Read the model definition and answer for the solid it produces. Units are mm, in the model's axes. A direction names the side the tool comes from. Coordinates: 2 decimals unless noted, no trailing zeros. Loops run counter-clockwise (first coordinate to the right, second up) from the corner with the lowest first, then second, coordinate; pieces in that order, holes last. Notation, with made-up numbers: M -38,8.25 L 5,8.25 A15 ccw 5,33.25 Z; hole C 30,85.25 d7. An arc over 180 degrees is marked long. Use one line per item in the form item = value. Start each with the question number.
1. For a pull along Z with two mould halves and no side action, classify faces 3 (the flat face through (0, 2, 8.334)), 4 (the cylindrical face through (0.628, 1.565, -14.274)), 5 (the flat face through (6, 0, 3)) as released by +Z, released by -Z, zero draft, split by the parting line, or undercut.
2. Find the intervals of material crossed by probe 1 along Z at (x, y) = (0.5, 0.3); probe 2 along X at (y, z) = (1.9, -5); probe 3 along X at (y, z) = (0.55, -0.25), in increasing order. Write a range as [from, to].
3. The part is cut by section B-B (z = -0.5). Give the vertices of the cut face in (x, y) (3 decimals), plus the area to 3 significant figures.
4. The part is cut by section D-D (x = 6.75). Give the vertices of the cut face in (y, z) (3 decimals), plus the area to 3 significant figures.
5. A tool of negligible diameter and unlimited length cuts with its end or side. For faces 1 (the flat face through (-1.191, 2, 7)), 2 (the flat face through (6, 3.175, 3)), from which of +Z, -Z, +X, -X, +Y, -Y can it reach the whole face along a straight path? Write none if from no direction.
6. The part is cut by section C-C (x = -4). Give the vertices of the cut face in (y, z) (3 decimals), plus the area to 3 significant figures.
7. The part is cut by section A-A (y = 0.65). Give the number of separate pieces and of enclosed holes in the cut face, plus the area to 3 significant figures.
8. A flat-ended cylindrical pin translates along its axis: pin 1 (1.7 mm diameter, centred on y = 1, z = 7, fed in from +X). Find the tip coordinate at first contact, or state that the pin passes through.
from build123d import *

# Parameters (mm, degrees)
SKETCH1_R           = 14.2875
BOSS_EXTRUDE2_DEPTH = 3.175


with BuildPart() as part:
    # Sketch1 → Boss-Extrude2 (new body)
    # profile 1 of 5: a face of its own
    with BuildSketch(Plane(origin=(0, 0, 0), x_dir=(1, 0, 0), z_dir=(0, 1, 0))):
        with Locations(Location((0, 0, 0), (0, 0, 270))):
            Circle(SKETCH1_R)
        with BuildLine():
            Line((-1.190625, 6.237380228), (-1.190625, 8.334375))
            Line((-1.190625, 8.334375), (1.190625, 8.334375))
            Line((1.190625, 8.334375), (1.190625, 6.237380228))
            ThreePointArc((1.190625, 6.237380228), (2.159427274, 5.971547023), (3.074180531, 5.55625))
            Line((3.074180531, 5.55625), (8.0362073, 5.55625))
            ThreePointArc((8.0362073, 5.55625), (9.6237073, 7.14375), (11.2112073, 5.55625))
            ThreePointArc((11.2112073, 5.55625), (10.4174573, 4.181434671), (8.8299573, 4.181434671))
            Line((8.8299573, 4.181434671), (6.348943915, -0.115806564))
            ThreePointArc((6.348943915, -0.115806564), (5.499261314, -3.175), (3.274763384, -5.440443436))
            Line((3.274763384, -5.440443436), (0.79375, -9.737684671))
            ThreePointArc((0.79375, -9.737684671), (1.374815329, -10.31875), (1.5875, -11.1125))
            ThreePointArc((1.5875, -11.1125), (-0.79375, -12.487315329), (-0.79375, -9.737684671))
            Line((-0.79375, -9.737684671), (-3.274763384, -5.440443436))
            ThreePointArc((-3.274763384, -5.440443436), (-5.499261314, -3.175), (-6.348943915, -0.115806564))
            Line((-6.348943915, -0.115806564), (-8.8299573, 4.181434671))
            ThreePointArc((-8.8299573, 4.181434671), (-10.998522628, 6.35), (-8.0362073, 5.55625))
            Line((-8.0362073, 5.55625), (-3.074180531, 5.55625))
            ThreePointArc((-3.074180531, 5.55625), (-2.159427274, 5.971547023), (-1.190625, 6.237380228))
        make_face(mode=Mode.SUBTRACT)
    # profile 2 of 5: a face of its own
    with BuildSketch(Plane(origin=(0, 0, 0), x_dir=(1, 0, 0), z_dir=(0, 1, 0))):
        with BuildLine():
            ThreePointArc((-6.348943915, -0.115806564), (-5.499261314, 3.175), (-3.074180531, 5.55625))
            Line((-3.074180531, 5.55625), (-8.0362073, 5.55625))
            ThreePointArc((-8.0362073, 5.55625), (-8.248891971, 4.7625), (-8.8299573, 4.181434671))
            Line((-8.8299573, 4.181434671), (-6.348943915, -0.115806564))
        make_face()
    # profile 3 of 5: a face of its own
    with BuildSketch(Plane(origin=(0, 0, 0), x_dir=(1, 0, 0), z_dir=(0, 1, 0))):
        with BuildLine():
            Line((8.0362073, 5.55625), (3.074180531, 5.55625))
            ThreePointArc((3.074180531, 5.55625), (5.470079815, 3.225015785), (6.35, 0))
            ThreePointArc((6.35, 0), (6.349735973, -0.05790569), (6.348943915, -0.115806564))
            Line((6.348943915, -0.115806564), (8.8299573, 4.181434671))
            ThreePointArc((8.8299573, 4.181434671), (8.248891971, 4.7625), (8.0362073, 5.55625))
        make_face()
    # profile 4 of 5: a face of its own
    with BuildSketch(Plane(origin=(0, 0, 0), x_dir=(1, 0, 0), z_dir=(0, 1, 0))):
        with BuildLine():
            Line((-1.190625, -8.334375), (-1.190625, -6.237380228))
            ThreePointArc((-1.190625, -6.237380228), (-2.267972755, -5.931171856), (-3.274763384, -5.440443436))
            Line((-3.274763384, -5.440443436), (-0.79375, -9.737684671))
            ThreePointArc((-0.79375, -9.737684671), (0, -9.525), (0.79375, -9.737684671))
            Line((0.79375, -9.737684671), (3.274763384, -5.440443436))
            ThreePointArc((3.274763384, -5.440443436), (2.267972755, -5.931171856), (1.190625, -6.237380228))
            Line((1.190625, -6.237380228), (1.190625, -8.334375))
            Line((1.190625, -8.334375), (-1.190625, -8.334375))
        make_face()
    # profile 5 of 5: a face of its own
    with BuildSketch(Plane(origin=(0, 0, 0), x_dir=(1, 0, 0), z_dir=(0, 1, 0))):
        with BuildLine():
            Line((1.190625, 8.334375), (-1.190625, 8.334375))
            Line((-1.190625, 8.334375), (-1.190625, 6.237380228))
            ThreePointArc((-1.190625, 6.237380228), (0, 6.35), (1.190625, 6.237380228))
            Line((1.190625, 6.237380228), (1.190625, 8.334375))
        make_face()
    extrude(amount=BOSS_EXTRUDE2_DEPTH)


solid = part.part
Computed values:
q1.face_3 = undercut
q1.face_4 = split by the parting line
q1.face_5 = zero draft
q2.probe_1 = [-14.28, -6.33], [8.33, 9.61], [12.62, 14.28]
q2.probe_2 = [-13.38, -11.11], [-8.14, -3.91], [3.91, 8.14], [11.11, 13.38]
q2.probe_3 = [-14.29, -6.35], [6.35, 14.29]
q3.outline = M -14.279,0 L -6.33,0 L -6.33,3.175 L -14.279,3.175 Z; M 6.33,0 L 14.279,0 L 14.279,3.175 L 6.33,3.175 Z
q3.area = 50.5 mm²
q4.outline = M 0,-12.592 L 3.175,-12.592 L 3.175,12.592 L 0,12.592 Z
q4.area = 80.0 mm²
q5.face_1 = +Y, -Y
q5.face_2 = +Z, -Z, +X, -X, +Y
q6.outline = M 0,-13.716 L 3.175,-13.716 L 3.175,-4.932 L 0,-4.932 Z; M 0,4.932 L 3.175,4.932 L 3.175,13.716 L 0,13.716 Z
q6.area = 55.8 mm²
q7.separate_pieces = 1
q7.enclosed_holes = 4
q7.area = 486 mm²
q8.pin_1 = 12.9
